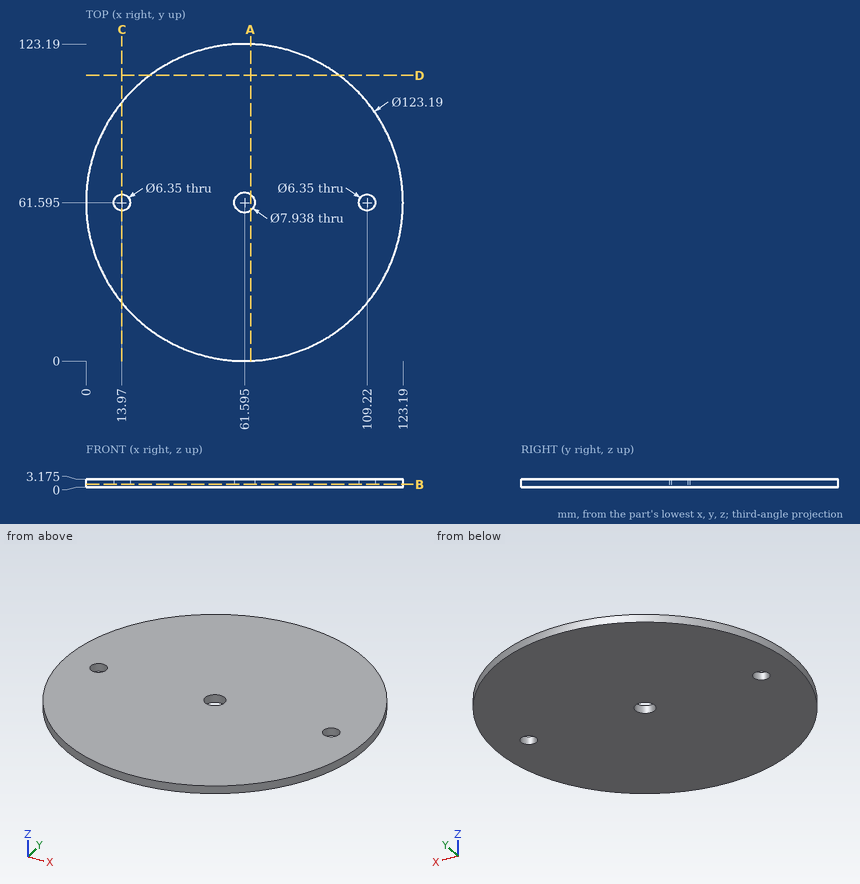
Could you check a few things on this drawing? It's one solid part, dimensions in mm from its lowest x, y, z. Coordinates: 2 decimals unless noted, no trailing zeros. Order: outer loops, then holes, each group sorted by start corner. A loop starts at its lowest first (then second) coordinate and runs counter-clockwise, first axis right, second up. Notation, with made-up numbers: (29.25, 25) - (50.25, 25) arc R23 cw to (50.25, 47) - close; hole circle Ø7 at (63, 70.25). An arc over 180 degrees is marked (long way). Answer as a JSON object with one key per item and string values. Group by question number.
Q1. Imagine slicing it at A-A (x = 64). Please give me the cut outline in (y, z) (1 decimal).
Q2. Will these pins go through, and if not, where does the flat tip stop? P1, Ø1, axis at x = 109.5, z = 1, coming from the +Y side (1 decimal); P2, Ø1.5, axis at y = 44, z = 2.5, coming from the -X side.
Q3. I need wall thicknesses on line 1 (X direction, y = 63.5, z = 2.45) (1 decimal); line 2 (Y direction, x = 61, z = 2.2); line 3 (Y direction, x = 109.22, z = 2.45) (1 decimal). Which ranges of each line are inside material? Lowest first, please. Write a range as from..to.
Q4. Imagine slicing it at B-B (z = 1.05). Give the number of separate pieces and of enclosed holes in the cut face, and give its area (3 significant figures).
Q5. Imagine slicing it at C-C (x = 13.97). Please give me the cut outline in (y, z) (1 decimal), and give its area (3 significant figures).
Q6. Imagine slicing it at D-D (y = 111). Please give me the cut outline in (x, z) (1 decimal).
Determined:
{
 "1": {"outline": "(0, 0) - (58.4, 0) - (58.4, 3.2) - (0, 3.2) - close; (64.8, 0) - (123.1, 0) - (123.1, 3.2) - (64.8, 3.2) - close"},
 "2": {"P1": "stops at y = 100.9", "P2": "stops at x = 2.35"},
 "3": {"line 1": "x = 0..11.4, 16.5..58.1, 65.1..106.7, 111.8..123.2", "line 2": "y = 0..57.67, 65.52..123.19", "line 3": "y = 22.5..58.4, 64.8..100.7"},
 "4": {"separate pieces": "1", "enclosed holes": "3", "area": "11,800 mm2"},
 "5": {"outline": "(22.5, 0) - (58.4, 0) - (58.4, 3.2) - (22.5, 3.2) - close; (64.8, 0) - (100.7, 0) - (100.7, 3.2) - (64.8, 3.2) - close", "area": "228 mm2"},
 "6": {"outline": "(24.8, 0) - (98.4, 0) - (98.4, 3.2) - (24.8, 3.2) - close"}
}
